Geometry: see drawing. Coordinates: mm, zero at the bounding-box minimum. A direction names the side the tool comes from. Give positions to 0.01 mm unless a question says otherwise; leave off trailing zeros. Loops run counter-clockwise (first coordinate to the right, second up) from the corner with the lowest first, then second, coordinate; pieces in that order, holes last. Notation, with made-up numbers: M 43.25,12.5 L 88.25,12.5 A27 ccw 88.25,45.5 Z; hole C -2.5,29.5 d8. An arc over 180 degrees is marked long. Answer in a Markdown table with one row per item.
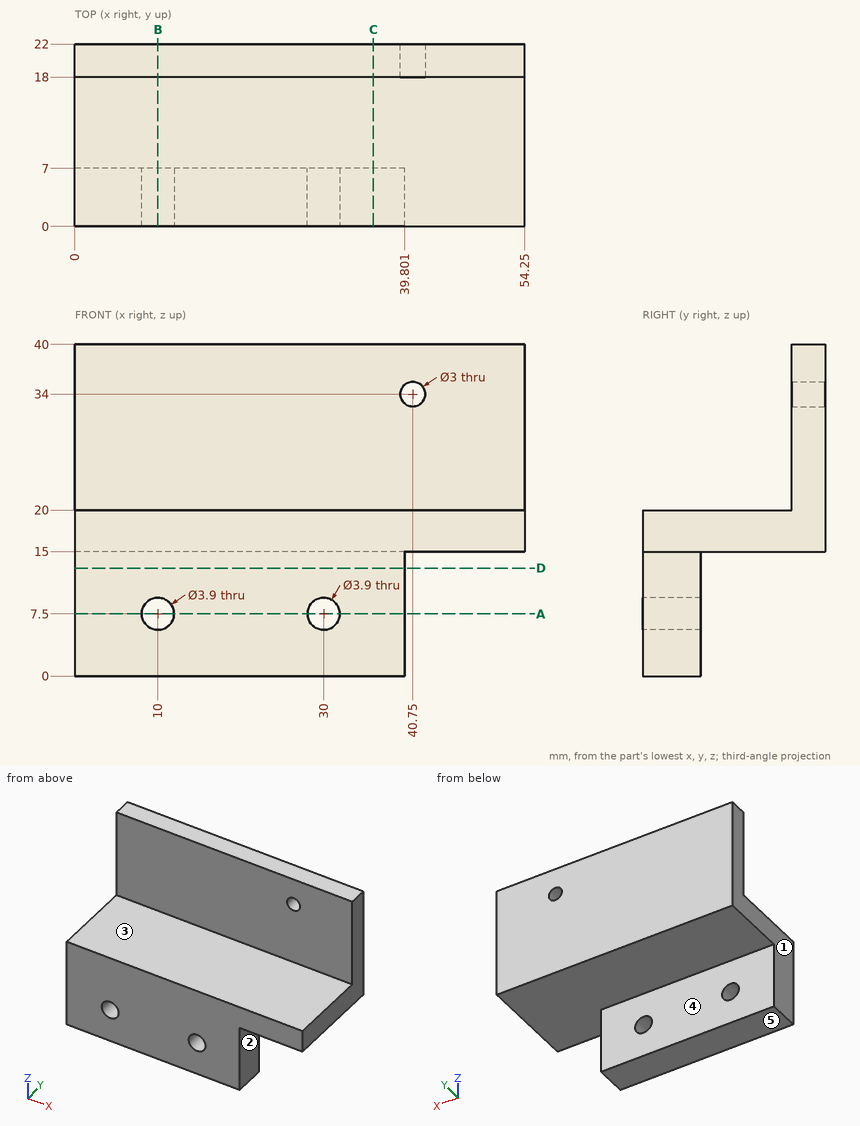
1) Set-up query: the marked faces 1, 2, 3, 4 and 5. Return all of +Z, -Z, +X, -X, +Y, -Y with unobstructed straight access to the full face (end or side cutting, diameter ignored); none if empty.
Reply:
| item | result |
|---|---|
| face 1 | +Z, -Z, -X, +Y, -Y |
| face 2 | -Z, +X, +Y, -Y |
| face 3 | +Z, +X, -X, -Y |
| face 4 | -Z, +X, -X, +Y |
| face 5 | -Z, +X, -X, +Y, -Y |
2) Pin query (flat end, axial travel): pin 1 Ø5 at (y, z) = (15, 26) entering from -X; pin 2 Ø3 at (x, y) = (14.5, 15.5) entering from +Z; pin 3 Ø16 at (x, z) = (22, 33.5) entering from -Y; pin 4 Ø4.5 at (x, z) = (30, 7.5) entering from +Y. Return the tip coordinate at first contact, or that it passes through.
Reply:
| item | result |
|---|---|
| pin 1 | passes through |
| pin 2 | stops at z = 20 |
| pin 3 | stops at y = 18 |
| pin 4 | stops at y = 7 |
3) Section D-D, the plane z = 13. Return loops of the section in (x, y), then the cut area to 3 significant figures.
Reply:
| item | result |
|---|---|
| outline | M 0,0 L 39.8,0 L 39.8,7 L 0,7 Z |
| area | 279 mm² |
4) Section B-B, the plane x = 10. Return loops of the section in (y, z).
Reply:
| item | result |
|---|---|
| outline | M 0,0 L 7,0 L 7,5.55 L 0,5.55 Z; M 0,9.45 L 7,9.45 L 7,15 L 22,15 L 22,40 L 18,40 L 18,20 L 0,20 Z |
5) Section A-A, the plane z = 7.5. Return loops of the section in (x, y), then the cut area to 3 significant figures.
Reply:
| item | result |
|---|---|
| outline | M 0,0 L 8.05,0 L 8.05,7 L 0,7 Z; M 11.95,0 L 28.05,0 L 28.05,7 L 11.95,7 Z; M 31.95,0 L 39.8,0 L 39.8,7 L 31.95,7 Z |
| area | 224 mm² |
6) Section C-C, the plane x = 36. Return loops of the section in (y, z).
Reply:
| item | result |
|---|---|
| outline | M 0,0 L 7,0 L 7,15 L 22,15 L 22,40 L 18,40 L 18,20 L 0,20 Z |
7) Material intervals for L1, parallel to X at y = 3, z = 7.5; L2, parallel to Z at x = 40.75, y = 20.3; L3, parallel to X at y = 19.05, z = 34, sorted ascending.
Reply:
| item | result |
|---|---|
| L1 | x = 0 to 8.05, 11.95 to 28.05, 31.95 to 39.8 |
| L2 | z = 15 to 32.5, 35.5 to 40 |
| L3 | x = 0 to 39.25, 42.25 to 54.25 |
